Can you work these out from the model? Positions are in its coordinate system, mm. Face numbers are marked on the shaded views. A direction names the side the tool comes from. Round coordinates to 2 decimals unless told otherwise and drop trailing zeros. Write each loop counter-clockwise with the first axis right and the second up, starting at its lowest first coordinate (ties: lowest second). Pieces come first, ordered by that corner, then holes. Notation, with made-up numbers: M -32.75,-36 L 22.25,-36 A6 cw 22.25,-27 Z; hole C 36,-21 d1. An arc over 180 degrees is marked long. Answer as a JSON object with one key per item and string values. Group by question number.
1) Suppose I cut it at A-A, the plane z = -2. Write out the boundary of the cut face in (x, y), and give its area (3 significant figures).
2) Suppose I cut it at C-C, the plane x = -14.25. Write out the boundary of the cut face in (y, z).
3) Suppose I cut it at D-D, the plane y = 3. Write out the boundary of the cut face in (x, z), and give its area (3 significant figures).
4) Suppose I cut it at B-B, the plane y = 14. Write out the boundary of the cut face in (x, z).
5) I'm going to push flat-ended pins straight in: pin 1 Ø12 at (x, z) = (-4, 2.5) entering from +Y; pin 2 Ø3 at (y, z) = (16, -8.5) entering from +X; pin 3 Ø6 at (x, y) = (2, 18.5) entering from -Z. Where does each tip first touch, or does it pass through?
6) On a 3-axis mill with a long thin cutter (end or side, diameter ignored), from which of +Z, -Z, +X, -X, +Y, -Y can I reach the whole of each face in a straight line? I mean the marked faces 4 and 5. Say none if no direction works.
7) Please list where these lines run through material, in increasing order: L1, parallel to Y at x = -12.85, z = -2; L2, parallel to Y at x = 2, z = 13.1; L3, parallel to Z at x = 8.75, y = 22.25. Write a range as [from, to].
8) If we mould it in two halves opening along Y, with no side actions, what happens to the marked faces 1, 2 and 3? For each: +Y half, -Y half, draft (parallel to the pull), parting line (faces both ways), or undercut.
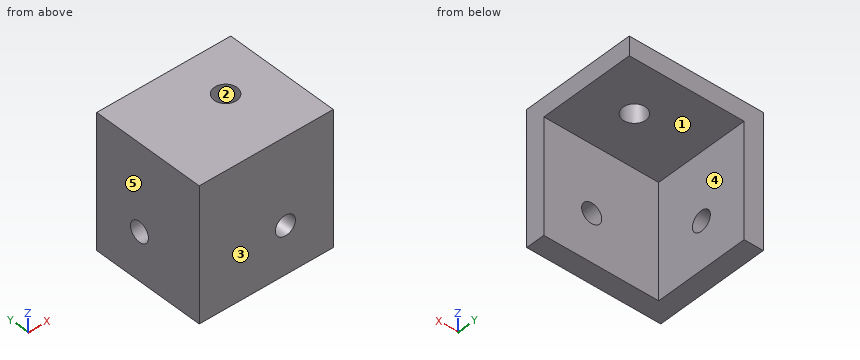
from build123d import *

# Parameters (mm, degrees)
SKETCH_1_W          = 24
SKETCH_1_H          = 24
SKETCH_1_R          = 2.1
EXTRUDE_1_DEPTH     = 4
EXTRUDE_2_DEPTH     = 24
SKETCH_2_R          = 2.379936998
CUT_EXTRUDE_1_DEPTH = 41.199502484
SKETCH_3_R          = 2.1
CUT_EXTRUDE_2_DEPTH = 41.199502484


with BuildPart() as part:
    # Sketch 1 → Extrude 1 (new body)
    with BuildSketch(Plane(origin=(0, 0, 0), x_dir=(1, 0, 0), z_dir=(0, 1, 0))):
        Rectangle(SKETCH_1_W, SKETCH_1_H)
        with Locations(Location((2, 2, 0), (0, 0, 270))):
            Circle(SKETCH_1_R, mode=Mode.SUBTRACT)
    extrude(amount=EXTRUDE_1_DEPTH)

    # Sketch 1_3 → Extrude 2 (add)
    with BuildSketch(Plane(origin=(0, 0, 0), x_dir=(1, 0, 0), z_dir=(0, 1, 0))):
        Polygon((-12, -12), (-12, 12), (-16, 12), (-16, -16), (12, -16), (12, -12), align=None)
    extrude(amount=EXTRUDE_2_DEPTH)

    # Sketch 2 → Cut-Extrude 1 (cut, through all)
    with BuildSketch(Plane.XY.offset(16)):
        with Locations((2, 14)):
            Circle(SKETCH_2_R)
    extrude(amount=-CUT_EXTRUDE_1_DEPTH, mode=Mode.SUBTRACT)

    # Sketch 3 → Cut-Extrude 2 (cut, through all)
    with BuildSketch(Plane.ZY.offset(16)):
        with Locations((-2, 14)):
            Circle(SKETCH_3_R)
    extrude(amount=-CUT_EXTRUDE_2_DEPTH, mode=Mode.SUBTRACT)


solid = part.part
Results:
{
 "1": {"outline": "M -16,0 L -0.1,0 L -0.1,4 L -12,4 L -12,11.9 L -16,11.9 Z; M -16,16.1 L -12,16.1 L -12,24 L -16,24 Z; M 4.1,0 L 12,0 L 12,4 L 4.1,4 Z", "area": "158 mm^2"},
 "2": {"outline": "M 0,-12 L 24,-12 L 24,16 L 0,16 Z; hole C 14,-2 d4.2"},
 "3": {"outline": "M -16,-12 L 12,-12 L 12,16 L -16,16 Z; hole C 2,-2 d4.2", "area": "770 mm^2"},
 "4": {"outline": "M -16,-12 L -12,-12 L -12,-4.1 L -16,-4.1 Z; M -16,0.1 L -12,0.1 L -12,12 L -0.38,12 L -0.38,16 L -16,16 Z; M 4.38,12 L 12,12 L 12,16 L 4.38,16 Z"},
 "5": {"pin 1": "y = 4", "pin 2": "x = -12", "pin 3": "z = 12"},
 "6": {"face 4": "-Z, +X, +Y", "face 5": "+Z, -Z, -X, +Y, -Y"},
 "7": {"L1": "[0, 11.9], [16.1, 24]", "L2": "[0, 11.62], [16.38, 24]", "L3": "[12, 16]"},
 "8": {"face 1": "draft", "face 2": "undercut", "face 3": "-Y half"}
}
